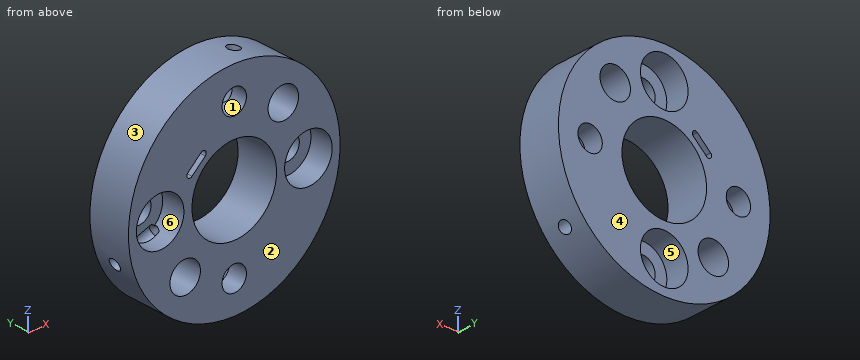
```python
from build123d import *

# Parameters (mm, degrees)
SKETCH1_R                                      = 15.875
BOSS_EXTRUDE1_DEPTH                            = 6.35
SKETCH2_R                                      = 6.35
CUT_EXTRUDE1_DEPTH                             = 24.3313898
CBORE_FOR_6_SOCKET_HEAD_CAP_SCREW1_D           = 3.6576
CBORE_FOR_6_SOCKET_HEAD_CAP_SCREW1_CBORE_D     = 7.14502
CBORE_FOR_6_SOCKET_HEAD_CAP_SCREW1_CBORE_DEPTH = 3.5052
CIRPATTERN1_COUNT                              = 2
SKETCH11_R                                     = 2.286
CUT_EXTRUDE2_DEPTH                             = 24.3313898
CIRPATTERN3_COUNT                              = 2
CIRPATTERN4_COUNT                              = 3
CUT_EXTRUDE3_DEPTH                             = 24.331389963
CBORE_FOR_6_SOCKET_HEAD_CAP_SCREW2_D           = 3.6576
CBORE_FOR_6_SOCKET_HEAD_CAP_SCREW2_CBORE_D     = 7.14502
CBORE_FOR_6_SOCKET_HEAD_CAP_SCREW2_CBORE_DEPTH = 3.5052
CIRPATTERN5_COUNT                              = 2


with BuildPart() as part:
    # Sketch1 → Boss-Extrude1 (new body)
    with BuildSketch(Plane(origin=(0, 0, 0), x_dir=(1, 0, 0), z_dir=(0, 1, 0))):
        with Locations(Location((0, 0, 0), (0, 0, 270))):
            Circle(SKETCH1_R)
    extrude(amount=BOSS_EXTRUDE1_DEPTH)

    # Sketch2 → Cut-Extrude1 (cut, through all)
    with BuildSketch(Plane(origin=(0, 6.35, 0), x_dir=(1, 0, 0), z_dir=(0, 1, 0))):
        with Locations(Location((0, 0, 0), (0, 0, 270))):
            Circle(SKETCH2_R)
    extrude(amount=-CUT_EXTRUDE1_DEPTH, mode=Mode.SUBTRACT)

    # CBORE for #6 Socket Head Cap Screw1 (through all)
    with Locations(Plane(origin=(0, 6.35, 0), x_dir=(1, 0, 0), z_dir=(0, 1, 0))):
        with Locations((0, 11.1252)):
            cbore_for_6_socket_head_cap_screw1 = CounterBoreHole(CBORE_FOR_6_SOCKET_HEAD_CAP_SCREW1_D / 2, CBORE_FOR_6_SOCKET_HEAD_CAP_SCREW1_CBORE_D / 2, CBORE_FOR_6_SOCKET_HEAD_CAP_SCREW1_CBORE_DEPTH)

    # CirPattern1: CBORE for #6 Socket Head Cap Screw1 ×2 about axis
    cirpattern1_axis = Axis((0, 0, 0), (0, 1, 0))
    for i in range(1, CIRPATTERN1_COUNT):
        add(cbore_for_6_socket_head_cap_screw1.rotate(cirpattern1_axis, i * 360 / CIRPATTERN1_COUNT), mode=Mode.SUBTRACT)

    # Sketch11 → Cut-Extrude2 (cut, through all)
    with BuildSketch(Plane(origin=(0, 6.35, 0), x_dir=(1, 0, 0), z_dir=(0, 1, 0))):
        with Locations(Location((-7.360856908, 8.324988999, 0), (0, 0, 270))):
            Circle(SKETCH11_R)
    cut_extrude2 = extrude(amount=-CUT_EXTRUDE2_DEPTH, mode=Mode.SUBTRACT)

    # CirPattern3: Cut-Extrude2 ×2 about axis
    cirpattern3_axis = Axis((0, 0, 0), (0, 1, 0))
    for i in range(1, CIRPATTERN3_COUNT):
        add(cut_extrude2.rotate(cirpattern3_axis, i * 360 / CIRPATTERN3_COUNT), mode=Mode.SUBTRACT)

    # Sketch16 → Tap Drill for #2-56 Tap3 (revolve, cut)
    with BuildSketch(Plane(origin=(12.093135875, 3.244987275, -10.284536436), x_dir=(-0.6478448148472237, 0, -0.7617723386127685), z_dir=(0, 1, 0))):
        Polygon((0, 0), (0, 7.095959572), (0.889, 6.35), (0.889, 0), align=None)
    tap_drill_for_2_56_tap3 = revolve(axis=Axis((16.930390226, 3.244987275, -14.39835101), (-0.7617723386127686, 0, 0.6478448148472237)), mode=Mode.SUBTRACT)

    # CirPattern4: Tap Drill for #2-56 Tap3 ×3 about axis
    cirpattern4_axis = Axis((0, 6.35, 0), (0, -1, 0))
    for i in range(1, CIRPATTERN4_COUNT):
        add(tap_drill_for_2_56_tap3.rotate(cirpattern4_axis, i * 360 / CIRPATTERN4_COUNT), mode=Mode.SUBTRACT)

    # Sketch17 → Cut-Extrude3 (cut, through all)
    with BuildSketch(Plane(origin=(0, 6.35, 0), x_dir=(1, 0, 0), z_dir=(0, 1, 0))):
        with BuildLine():
            Line((-4.96914615, -6.489934512), (-6.955810814, -4.646503161))
            ThreePointArc((-6.955810814, -4.646503161), (-6.979764598, -4.005972756), (-6.339234193, -3.982018972))
            Line((-6.339234193, -3.982018972), (-4.352569529, -5.825450323))
            ThreePointArc((-4.352569529, -5.825450323), (-4.328615745, -6.465980728), (-4.96914615, -6.489934512))
        make_face()
    extrude(amount=-CUT_EXTRUDE3_DEPTH, mode=Mode.SUBTRACT)

    # CBORE for #6 Socket Head Cap Screw2 (through all)
    with Locations(Plane(origin=(11.1252, 0, 0), x_dir=(0, 0, -1), z_dir=(0, -1, 0))):
        with Locations((0, 0)):
            cbore_for_6_socket_head_cap_screw2 = CounterBoreHole(CBORE_FOR_6_SOCKET_HEAD_CAP_SCREW2_D / 2, CBORE_FOR_6_SOCKET_HEAD_CAP_SCREW2_CBORE_D / 2, CBORE_FOR_6_SOCKET_HEAD_CAP_SCREW2_CBORE_DEPTH)

    # CirPattern5: CBORE for #6 Socket Head Cap Screw2 ×2 about axis
    cirpattern5_axis = Axis((0, 0, 0), (0, 1, 0))
    for i in range(1, CIRPATTERN5_COUNT):
        add(cbore_for_6_socket_head_cap_screw2.rotate(cirpattern5_axis, i * 360 / CIRPATTERN5_COUNT), mode=Mode.SUBTRACT)


solid = part.part
```
CAD build for the part. Positions are in the model's coordinates, mm. Face numbers are marked on the shaded views. A direction names the side the tool comes from. Round coordinates to 2 decimals unless told otherwise and drop trailing zeros. Write each loop counter-clockwise with the first axis right and the second up, starting at its lowest first coordinate (ties: lowest second). Pieces come first, ordered by that corner, then holes. Notation, with made-up numbers: M -37.75,61 L -29.75,61 A24 ccw -29.75,88 Z; hole C -36.75,71 d7. An arc over 180 degrees is marked long. One line per question, with ' | ' between items.
1. Pin check, flat tips, straight feed: pin 1 Ø1.5 at (x, y) = (11.5, 2) entering from -Z; pin 2 Ø5 at (x, z) = (0, -11.13) entering from +Y; pin 3 Ø3 at (x, z) = (0, 11.13) entering from -Y; pin 4 Ø1 at (y, z) = (5.5, 5.5) entering from -X. Stop position of each tip, or through.
Working result:
pin 1: z = -11.68 | pin 2: y = 2.84 | pin 3: through | pin 4: x = -15.07
2. Which spindle directions (+Z, -Z, +X, -X, +Y, -Y) get a long thin tool onto all of the face, cutting with end or side? Do the marked faces 4, 5 and 6. Say none if no direction does.
Working result:
face 4: +Z, -Z, +X, -X, +Y | face 5: +Y | face 6: -Y
3. Cut at C-C on y = 5.5. Count the separate pieces of the cut face and the enclosed holes in it, and give its area (3 significant figures).
Working result:
separate pieces: 1 | enclosed holes: 8 | area: 528 mm2
4. Cut at A-A on x = 0. Write the cut outline in (y, z) (3 decimals).
Working result:
outline: M 0,-15.875 L 6.35,-15.875 L 6.35,-14.698 L 2.845,-14.698 L 2.845,-12.954 L 0,-12.954 Z; M 0,-9.296 L 2.845,-9.296 L 2.845,-7.553 L 6.35,-7.553 L 6.35,-6.35 L 0,-6.35 Z; M 0,6.35 L 6.35,6.35 L 6.35,7.553 L 2.845,7.553 L 2.845,9.296 L 0,9.296 Z; M 0,12.954 L 2.845,12.954 L 2.845,14.698 L 6.35,14.698 L 6.35,15.875 L 0,15.875 Z
5. Mould opens along X. For the marked faces 1, 2 and 3 say: pulls with the +X half, pulls with the -X half, needs draft (parallel to the pull), parting line crosses it, or undercut.
Working result:
face 1: undercut | face 2: needs draft | face 3: parting line crosses it
6. Probe L1, parallel to X at y = 3.25, z = 0 (3 decimals); L2, parallel to X at y = 1.5, z = 9.5; L3, parallel to X at y = 2.25, z = 4.5. List the from-to ranges inside material, lowest first. Write a range as from..to.
Working result:
L1: -15.875..-14.698, -7.553..-6.35, 6.35..7.553, 14.698..15.875 | L2: -12.72..-0.84, 0.84..5.4, 9.32..12.72 | L3: -15.22..-7.06, -5.78..-4.48, 4.48..15.22
7. Cut at D-D on x = -5.5. Write the cut outline in (y, z), and give its area (3 significant figures).
Working result:
outline: M 0,-14.89 L 6.35,-14.89 L 6.35,-9.65 L 0,-9.65 Z; M 0,-7 L 6.35,-7 L 6.35,-3.17 L 0,-3.17 Z; M 0,3.17 L 6.35,3.17 L 6.35,4.76 L 0,4.76 Z; M 0,6 L 6.35,6 L 6.35,14.89 L 0,14.89 Z | area: 124 mm2
8. Cut at B-B on z = 0. Write the cut outline in (x, y) (3 decimals), and give its area (3 significant figures).
Working result:
outline: M -15.875,0 L -14.698,0 L -14.698,3.505 L -12.954,3.505 L -12.954,6.35 L -15.875,6.35 Z; M -9.296,3.505 L -7.553,3.505 L -7.553,0 L -6.35,0 L -6.35,6.35 L -9.296,6.35 Z; M 6.35,0 L 7.553,0 L 7.553,3.505 L 9.296,3.505 L 9.296,6.35 L 6.35,6.35 Z; M 12.954,3.505 L 14.698,3.505 L 14.698,0 L 15.875,0 L 15.875,6.35 L 12.954,6.35 Z | area: 50.1 mm2
